from build123d import *

# Parameters (mm, degrees)
SKETCH_1_R      = 1.6
EXTRUDE_1_DEPTH = 2


with BuildPart() as part:
    # ｽｹｯﾁ1 → ﾎﾞｽ - 押し出し1 (new body)
    with BuildSketch(Plane.XY):
        with BuildLine():
            Line((20, 0), (50, 0))
            Line((50, 0), (50, 10))
            Line((50, 10), (60, 10))
            ThreePointArc((60, 10), (43.011626335, 43.011626335), (10, 60))
            Line((10, 60), (10, 50))
            Line((10, 50), (0, 50))
            Line((0, 50), (0, 10))
            Line((0, 10), (20, 10))
            Line((20, 10), (20, 0))
        make_face()
        with Locations((5, 35)):
            Circle(SKETCH_1_R, mode=Mode.SUBTRACT)
        with Locations((5, 15)):
            Circle(SKETCH_1_R, mode=Mode.SUBTRACT)
        with Locations((25, 5)):
            Circle(SKETCH_1_R, mode=Mode.SUBTRACT)
        with Locations((45, 5)):
            Circle(SKETCH_1_R, mode=Mode.SUBTRACT)
    extrude(amount=EXTRUDE_1_DEPTH)


solid = part.part
Can you work these out from the model? Positions are in its coordinate system, mm. A direction names the side the tool comes from. Round coordinates to 2 decimals unless told otherwise and drop trailing zeros. Write each loop counter-clockwise with the first axis right and the second up, starting at its lowest first coordinate (ties: lowest second). Pieces come first, ordered by that corner, then holes. Notation, with made-up numbers: M -36,-3.5 L -20,-3.5 A20 cw -20,3.5 Z; hole C -24.75,1.5 d3. An arc over 180 degrees is marked long. Use CSV: the item, a comma, the result in double quotes.
(1) Imagine slicing it at D-D (y = 15). Write out the boundary of the cut face in (x, z).
Check values:
outline,"M 0,0 L 3.4,0 L 3.4,2 L 0,2 Z; M 6.6,0 L 58.95,0 L 58.95,2 L 6.6,2 Z"
(2) I'm going to push flat-ended pins straight in: pin 1 (1 mm diameter, centred on x = 4.5, z = 1, fed in from +Y); pin 2 (0.6 mm diameter, centred on x = 6.5, z = 0.5, fed in from -Y); pin 3 (1 mm diameter, centred on x = 30, z = 1.5, fed in from +Y). Where does each tip first touch, or does it pass through?
Check values:
pin 1,"y = 50"
pin 2,"y = 10"
pin 3,"y = 53.2"
(3) We'd pull the mould along X, two halves only. Please class faces 1 (the flat face through (0, 30, 1)), 2 (the cylindrical face through (4.792, 16.586, 0.986)), 3 (the flat face through (10, 10, 1)): +X half, -X half, draft (parallel to the pull), parting line (faces both ways), or undercut.
Check values:
face 1,"-X half"
face 2,"undercut"
face 3,"draft"
(4) On a 3-axis mill with a long thin cutter (end or side, diameter ignored), from which of +Z, -Z, +X, -X, +Y, -Y can I reach the whole of each face in a straight line? I mean faces 4 (the flat face through (5, 50, 1)), 5 (the flat face through (50, 5, 1)), 6 (the flat face through (20, 5, 1)), 7 (the flat face through (30, 24, 2)). Say none if no direction works.
Check values:
face 4,"+Z, -Z, -X, +Y"
face 5,"+Z, -Z, +X, -Y"
face 6,"+Z, -Z, -X, -Y"
face 7,"+Z, +X, -X, +Y, -Y"
(5) I need wall thicknesses on line 1 along Y through (x, z) = (5, 1); line 2 along X through (y, z) = (15.5, 0.2); line 3 along Y through (x, z) = (9, 0.6). Which ranges of each line are inside material? Lowest first, please.
Check values:
line 1,"10 to 13.4, 16.6 to 33.4, 36.6 to 50"
line 2,"0 to 3.48, 6.52 to 58.82"
line 3,"10 to 50"
(6) Imagine slicing it at C-C (y = 5). Write out the boundary of the cut face in (x, z).
Check values:
outline,"M 20,0 L 23.4,0 L 23.4,2 L 20,2 Z; M 26.6,0 L 43.4,0 L 43.4,2 L 26.6,2 Z; M 46.6,0 L 50,0 L 50,2 L 46.6,2 Z"
(7) Imagine slicing it at A-A (z = 0.9). Write out the boundary of the cut face in (x, y), plus the area to 3 significant figures.
Check values:
outline,"M 0,10 L 20,10 L 20,0 L 50,0 L 50,10 L 60,10 A60.83 ccw 10,60 L 10,50 L 0,50 Z; hole C 5,15 d3.2; hole C 5,35 d3.2; hole C 25,5 d3.2; hole C 45,5 d3.2"
area,"2,460 mm^2"
(8) Imagine slicing it at B-B (x = 5). Write out the boundary of the cut face in (y, z).
Check values:
outline,"M 10,0 L 13.4,0 L 13.4,2 L 10,2 Z; M 16.6,0 L 33.4,0 L 33.4,2 L 16.6,2 Z; M 36.6,0 L 50,0 L 50,2 L 36.6,2 Z"
